Autodesk Inventor part; units mm, degrees
ref_plane "YZ Plane" through (0, 0, 0) normal (1, 0, 0) x (0, 1, 0)
ref_plane "XZ Plane" through (0, 0, 0) normal (0, 1, 0) x (-1, 0, 0)
ref_plane "XY Plane" through (0, 0, 0) normal (0, 0, 1) x (1, 0, 0)
ref_plane "Work Plane1" through (52.5141, 202.7033, 6.4479) normal (0, 0, -1) x (0, 1, 0)
sketch "Sketch1" plane through (52.5141, 202.7033, 6.4479) normal (0, 0, -1) x (0, 1, 0)
  circle A0 centre (-59.8114, -30.5) radius 1.4 construction
  circle A1 centre (-38.8114, -18.3756) radius 1.4
  circle A2 centre (-38.8114, -42.6244) radius 1.4 construction
  circle A3 centre (41, 0) radius 1.65
  circle A4 centre (-9, 0) radius 1.65
  circle A5 centre (-9, 50) radius 1.65
  circle A6 centre (41, 50) radius 1.65
  circle A7 centre (16, 50) radius 1.65
  circle A8 centre (-9, 25) radius 1.65
  circle A9 centre (16, 0) radius 1.65
  circle A10 centre (41, 25) radius 1.65
  line L0 (80, 55) -> (-80, 55)
  line L1 (-80, 55) -> (-80, -55)
  line L2 (-80, -55) -> (80, -55)
  line L3 (80, -55) -> (80, 55)
  line L4 (-36.5, 0) -> (-36.5, -50)
  line L5 (-14, 0) -> (-36.5, 0)
  line L6 (-14, -5) -> (-14, 0)
  line L7 (72, -5) -> (-14, -5)
  line L8 (72, -50) -> (72, -5)
  line L9 (-36.5, -50) -> (72, -50)
  line L10 (-4, 45) -> (-4, 5)
  line L11 (36, 45) -> (-4, 45)
  line L12 (36, 5) -> (36, 45)
  line L13 (-4, 5) -> (36, 5)
  line L14 (-64.5989, -17.0433) -> (-64.5989, -57.0433) construction
  line L15 (-64.5989, -57.0433) -> (-34.5989, -57.0433) construction
  line L16 (-34.5989, -57.0433) -> (-34.5989, -17.0433) construction
  line L17 (-34.5989, -17.0433) -> (-64.5989, -17.0433) construction
  line L18 (-34.8114, -13.0433) -> (-63.8114, -13.0433)
  line L19 (-63.8114, -13.0433) -> (-63.8114, -52.6244)
  line L20 (-63.8114, -52.6244) -> (-34.8114, -52.6244)
  line L21 (-34.8114, -52.6244) -> (-34.8114, -13.0433)
  circle A11 centre (-59.8114, -30.5) radius 2.95
  circle A12 centre (-38.8114, -18.3756) radius 2.95
  circle A13 centre (-38.8114, -42.6244) radius 2.95 construction
  line L22 (-36.5, -35.1157) -> (-41.75, -35.1157) construction
  line L23 (-41.75, -35.1157) -> (-41.75, -38.5657) construction
  line L24 (-41.75, -38.5657) -> (-56.86, -38.5657) construction
  line L25 (-56.86, -38.5657) -> (-56.86, -35.1157) construction
  line L26 (-56.86, -35.1157) -> (-60.26, -35.1157) construction
  line L27 (-60.26, -35.1157) -> (-60.26, -52.0657) construction
  line L28 (-60.26, -52.0657) -> (-36.5, -52.0657) construction
  line L29 (-36.5, -52.0657) -> (-36.5, -35.1157) construction
  line L30 (-41.75, -28.3657) -> (-36.5, -28.3657) construction
  line L31 (-36.5, -28.3657) -> (-36.5, -25.0657) construction
  line L32 (-36.5, -25.0657) -> (-60.26, -25.0657) construction
  line L33 (-60.26, -25.0657) -> (-60.26, -28.3657) construction
  line L34 (-60.26, -28.3657) -> (-56.86, -28.3657) construction
  line L35 (-56.86, -28.3657) -> (-56.86, -27.0942) construction
  line L36 (-56.86, -27.0942) -> (-41.75, -27.0942) construction
  line L37 (-41.75, -27.0942) -> (-41.75, -28.3657) construction
  line L38 (-56.86, -35.1157) -> (-60.26, -35.1157) construction
  line L39 (-56.86, -38.5657) -> (-56.86, -35.1157) construction
  line L40 (-41.75, -38.5657) -> (-56.86, -38.5657) construction
  line L41 (-41.75, -35.1157) -> (-41.75, -38.5657) construction
  line L42 (-36.5, -35.1157) -> (-41.75, -35.1157) construction
  line L43 (-36.5, -35.05) -> (-36.5, -35.1157) construction
  line L44 (-36.5, -35.05) -> (-56.86, -35.05) construction
  line L45 (-36.5, -34.78) -> (-36.5, -35.05) construction
  line L46 (-36.5, -34.78) -> (-56.86, -34.78) construction
  line L47 (-36.5, -34.51) -> (-36.5, -34.78) construction
  line L48 (-36.5, -34.51) -> (-56.86, -34.51) construction
  line L49 (-36.5, -34.24) -> (-36.5, -34.51) construction
  line L50 (-36.5, -34.24) -> (-56.86, -34.24) construction
  line L51 (-36.5, -33.97) -> (-36.5, -34.24) construction
  line L52 (-36.5, -33.97) -> (-56.86, -33.97) construction
  line L53 (-36.5, -33.7) -> (-36.5, -33.97) construction
  line L54 (-36.5, -33.7) -> (-56.86, -33.7) construction
  line L55 (-36.5, -33.43) -> (-36.5, -33.7) construction
  line L56 (-36.5, -33.43) -> (-56.86, -33.43) construction
  line L57 (-36.5, -33.16) -> (-36.5, -33.43) construction
  line L58 (-36.5, -33.16) -> (-56.86, -33.16) construction
  line L59 (-36.5, -32.89) -> (-36.5, -33.16) construction
  line L60 (-36.5, -32.89) -> (-56.86, -32.89) construction
  line L61 (-36.5, -32.62) -> (-36.5, -32.89) construction
  line L62 (-36.5, -32.62) -> (-56.86, -32.62) construction
  line L63 (-36.5, -32.35) -> (-36.5, -32.62) construction
  line L64 (-36.5, -32.35) -> (-56.86, -32.35) construction
  line L65 (-36.5, -32.08) -> (-36.5, -32.35) construction
  line L66 (-36.5, -32.08) -> (-56.86, -32.08) construction
  line L67 (-36.5, -31.81) -> (-36.5, -32.08) construction
  line L68 (-36.5, -31.81) -> (-56.86, -31.81) construction
  line L69 (-36.5, -31.54) -> (-36.5, -31.81) construction
  line L70 (-36.5, -31.54) -> (-56.86, -31.54) construction
  line L71 (-36.5, -31.27) -> (-36.5, -31.54) construction
  line L72 (-36.5, -31.27) -> (-56.86, -31.27) construction
  line L73 (-36.5, -31) -> (-36.5, -31.27) construction
  line L74 (-36.5, -31) -> (-56.86, -31) construction
  line L75 (-36.5, -30.73) -> (-36.5, -31) construction
  line L76 (-36.5, -30.73) -> (-56.86, -30.73) construction
  line L77 (-36.5, -30.46) -> (-36.5, -30.73) construction
  line L78 (-36.5, -30.46) -> (-56.86, -30.46) construction
  line L79 (-36.5, -30.19) -> (-36.5, -30.46) construction
  line L80 (-36.5, -30.19) -> (-56.86, -30.19) construction
  line L81 (-36.5, -29.92) -> (-36.5, -30.19) construction
  line L82 (-36.5, -29.92) -> (-56.86, -29.92) construction
  line L83 (-36.5, -29.65) -> (-36.5, -29.92) construction
  line L84 (-36.5, -29.65) -> (-56.86, -29.65) construction
  line L85 (-36.5, -29.38) -> (-36.5, -29.65) construction
  line L86 (-36.5, -29.38) -> (-56.86, -29.38) construction
  line L87 (-36.5, -29.11) -> (-36.5, -29.38) construction
  line L88 (-36.5, -29.11) -> (-56.86, -29.11) construction
  line L89 (-36.5, -28.84) -> (-36.5, -29.11) construction
  line L90 (-36.5, -28.84) -> (-56.86, -28.84) construction
  line L91 (-36.5, -28.3657) -> (-36.5, -28.84) construction
  line L92 (-41.75, -28.3657) -> (-36.5, -28.3657) construction
  line L93 (-41.75, -27.0942) -> (-41.75, -28.3657) construction
  line L94 (-56.86, -27.0942) -> (-41.75, -27.0942) construction
  line L95 (-56.86, -28.3657) -> (-56.86, -27.0942) construction
  line L96 (-60.26, -28.3657) -> (-56.86, -28.3657) construction
  line L97 (-60.26, -35.1157) -> (-60.26, -28.3657) construction
  line L98 (-60.26, -25.0657) -> (-36.5, -25.0657) construction
  line L99 (-36.5, -25.0657) -> (-36.5, -52.0657) construction
  line L100 (-60.26, -52.0657) -> (-60.26, -25.0657) construction
  line L101 (-57.1632, -22.5233) -> (-33.4032, -22.5233) construction
  line L102 (-33.4032, -22.5233) -> (-33.4032, -49.5233) construction
  line L103 (-33.4032, -49.5233) -> (-57.1632, -49.5233) construction
  line L104 (-57.1632, -49.5233) -> (-57.1632, -22.5233) construction
  circle A14 centre (-38.8114, -42.6244) radius 2.95
  point P0 (-202.7033, -52.5141)
  point P1 (-56.7146, -27.9576)
  dimension "d0" = 4
  dimension "d2" = 4
  dimension "d3" = 4
  dimension "d4" = 5.9
  dimension "d5" = 5.9
  dimension "d6" = 5.9
  dimension "d10" = 10
extrude "Extrusion1" add sketch "Sketch1" along normal blind 4 contours L18 L21 L9 L4 A14 A12 | L4 A12 A14 L9 L21 L20 L19 L18
sketch "Sketch2" plane through (52.5141, 202.7033, 2.4479) normal (0, 0, -1) x (-1, 0, 0)
  circle A0 centre (42.6244, -38.8114) radius 2.95
  circle A1 centre (18.3756, -38.8114) radius 2.95
  circle A2 centre (30.5, -59.8114) radius 2.95
  line L0 (13.0433, -34.8114) -> (13.0433, -63.8114)
  line L1 (13.0433, -63.8114) -> (52.6244, -63.8114)
  line L2 (52.6244, -63.8114) -> (52.6244, -34.8114)
  line L3 (52.6244, -34.8114) -> (13.0433, -34.8114)
  point P0 (52.5141, -202.7033)
extrude "Extrusion2" add sketch "Sketch2" along normal blind 1.5 contours A0 | A1 | A2 | L3 L2 L1 L0
sketch "Sketch3" plane through (-0.1103, 138.8919, 6.4479) normal (0, -1, 0) x (1, 0, 0)
  line L0 (39.581, 0) -> (0, 0)
  line L1 (0, 0) -> (0, -5.5)
  line L2 (39.581, -5.5) -> (0, -5.5)
  line L3 (39.581, 0) -> (39.581, -5.5)
  line L4 (17.5087, -7.4479) -> (17.5087, -6.8479) construction
  line L5 (17.5087, -6.8479) -> (24.2587, -6.8479) construction
  line L6 (24.2587, -6.8479) -> (24.2587, -7.4479) construction
  line L7 (27.5587, -7.4479) -> (24.2587, -7.4479) construction
  line L8 (27.5587, -6.4479) -> (27.5587, -7.4479) construction
  line L9 (27.5587, -6.4479) -> (0.5587, -6.4479) construction
  line L10 (0.5587, -6.4479) -> (0.5587, -7.4479) construction
  line L11 (17.5087, -7.4479) -> (0.5587, -7.4479) construction
  line L12 (39.581, 0) -> (39.581, -5.5)
  line L13 (39.581, -5.5) -> (34.8694, -5.5)
  line L14 (34.8694, -5.5) -> (34.8694, -6)
  line L15 (34.8694, -6.8) -> (39.581, -6.8)
  line L16 (39.581, -6.8) -> (39.581, -5.5)
  line L17 (39.581, -6.8) -> (32.6714, -6.8)
  line L18 (32.6714, -6.8) -> (34.8694, -6)
  line L19 (12.6726, -5.5) -> (12.6726, -6.5)
  line L20 (0, 0) -> (0, -5.5)
  line L21 (0, -5.5) -> (8.1109, -5.5)
  line L22 (8.1109, -6.8) -> (0, -6.8)
  line L23 (0, -6.8) -> (0, -5.5)
  line L24 (9.7457, -6.8) -> (8.1109, -6.8)
  line L25 (0, -5.5) -> (39.581, -5.5)
  line L26 (9.7457, -6.8) -> (7.5477, -6)
  line L27 (7.5477, -6) -> (7.5477, -5.5)
  line L28 (8.8457, -5.5) -> (33.4957, -5.5) construction
  line L29 (33.4957, -5.5) -> (33.4957, -6.5) construction
  line L30 (33.4957, -6.5) -> (8.8457, -6.5) construction
  line L31 (8.8457, -6.5) -> (8.8457, -5.5) construction
  point P0 (8.981, -5.5)
  dimension "d42" = 1.3
  dimension "d43" = 110
  dimension "d45" = 0.5
  dimension "d46" = 0.5
  dimension "d47" = 110
  dimension "d48" = 24.65
  dimension "d49" = 1
  dimension "d50" = 0.9
  dimension "d51" = 0
extrude "Extrusion3" add sketch "Sketch3" against normal up to surface (29 mm away) contours L16 L15 L17 L18 L14 L2 | L2 L27 L26 L24 L22 L23
sketch "Sketch6" plane through (52.5141, 202.7033, 6.4479) normal (0, 0, 1) x (1, 0, 0)
  line L0 (-13.0433, -34.8114) -> (-13.0433, -63.8114)
  line L1 (-52.6244, -34.8114) -> (-13.0433, -34.8114)
  line L2 (-52.6244, -63.8114) -> (-52.6244, -34.8114)
  line L3 (-13.0433, -63.8114) -> (-52.6244, -63.8114)
  line L4 (-23.5962, -45.8071) -> (-17.5454, -39.7563)
  line L5 (-17.5454, -39.7563) -> (-19.6668, -37.635)
  line L6 (-19.6668, -37.635) -> (-25.7175, -43.6858)
  line L7 (-25.7175, -43.6858) -> (-23.5962, -45.8071)
  line L8 (-23.5962, -45.8071) -> (-19.6668, -37.635) construction
  line L9 (-17.5454, -39.7563) -> (-25.7175, -43.6858) construction
  line L10 (-39.0797, -45.8071) -> (-43.9064, -40.9803)
  line L11 (-43.9064, -40.9803) -> (-41.7851, -38.859)
  line L12 (-41.7851, -38.859) -> (-36.9583, -43.6858)
  line L13 (-36.9583, -43.6858) -> (-39.0797, -45.8071)
  line L14 (-39.0797, -45.8071) -> (-41.7851, -38.859) construction
  line L15 (-43.9064, -40.9803) -> (-36.9583, -43.6858) construction
  line L16 (-25.7175, -43.6858) -> (-36.9583, -43.6858)
  line L17 (-23.5962, -45.8071) -> (-23.5962, -49.9899)
  line L18 (-23.5962, -49.9899) -> (-39.0797, -49.9899)
  line L19 (-39.0797, -49.9899) -> (-39.0797, -45.8071)
  point P0 (-52.5141, -202.7033)
  point P1 (-21.6315, -41.7211)
  point P2 (-40.4324, -42.333)
  dimension "d35" = 3
  dimension "d36" = 3
  dimension "d37" = 45
  dimension "d38" = 0
extrude "Extrusion6" [suppressed]
properties part number "cellSTORM_v5_chiptray_new_0_24.4"
Verification items for the finished model (mm, model axes). A direction names the side the tool comes from. Coordinates: 2 decimals unless noted, no trailing zeros. Order: outer loops, then holes, each group sorted by start corner. A loop starts at its lowest first (then second) coordinate and runs counter-clockwise, first axis right, second up. Notation, with made-up numbers: (-22.75, 52) -> (25.25, 52) arc R21 ccw to (25.25, 57) -> close; hole circle Ø11 at (-31.75, 70.25). An arc over 180 degrees is marked (long way). Answer as CSV lines item,"result". Start each with the question number.
1) Material ranges on L1, parallel to X at y = 160, z = 0.5; L2, parallel to X at y = 162.5, z = 3.5; L3, parallel to X at y = 163.5, z = 3.5, recorded low to high. Write a range as [from, to].
2) Set-up check for faces 4 (the face through (5, 153, -0.352)), 5 (the face through (34, 164, 2.448)), 6 (the face through (33.64, 153.19, 0.04)): record each of +Z, -Z, +X, -X, +Y, -Y from which the full face is reachable in a straight line by a thin tool's end or side.
3) Gauge pin test, flat ends, axial feed: pin 1 Ø5.5 at (x, y) = (22.01, 142.89) entering from -Z; pin 2 Ø1.8 at (x, y) = (22, 141.5) entering from +Z. Record the tip position at first contact, or that the pin passes through.
4) Cross-section at B-B, the plane x = 24. Record the boundary of the cut face in (y, z), then the cut area to 3 significant figures.
5) Release check for a two-part mould opening along X. For faces 1 (the face through (39.471, 154, 4)), 2 (the face through (36, 153, -0.352)), 3 (the face through (22, 143, 2.448)) record: released by +X, released by -X, zero draft, split by the parting line, or undercut.
6) Cross-section at C-C, the plane z = 3.5. Record the boundary of the cut face in (x, y), then the cut area to 3 significant figures.
Conclusion:
1,L1,"x = [-0.11, 7.44], [34.76, 39.47]"
1,L2,"x = [-0.11, 7.29], [12.49, 31.54], [36.74, 39.47]"
1,L3,"x = [-0.11, 6.97], [12.81, 31.21], [37.06, 39.47]"
2,face 4,"-Z, +X, -X, +Y, -Y"
2,face 5,"+Z"
2,face 6,"+Y, -Y"
3,pin 1,"stops at z = 0.95"
3,pin 2,"stops at z = 2.45"
4,outline,"(138.89, 0.95) -> (167.89, 0.95) -> (167.89, 6.45) -> (145.07, 6.45) -> (145.07, 2.45) -> (140.71, 2.45) -> (140.71, 6.45) -> (138.89, 6.45) -> close"
4,area,"142 mm²"
5,face 1,"released by +X"
5,face 2,"zero draft"
5,face 3,"undercut"
6,outline,"(-0.11, 138.89) -> (39.47, 138.89) -> (39.47, 167.89) -> (-0.11, 167.89) -> close; hole circle Ø5.9 at (9.89, 163.89); hole circle Ø5.9 at (22.01, 142.89); hole circle Ø5.9 at (34.14, 163.89)"
6,area,"1,070 mm²"
